CAD build for the part. Positions are in the model's coordinates, mm. A direction names the side the tool comes from. Round coordinates to 2 decimals unless told otherwise and drop trailing zeros. Loops run counter-clockwise (first coordinate to the right, second up) from the corner with the lowest first, then second, coordinate; pieces in that order, holes last. Notation, with made-up numbers: (57, 13.5) - (67, 13.5) arc R27 ccw to (67, 31.5) - close; hole circle Ø8 at (53, 4.5). An arc over 180 degrees is marked (long way). Use one line per item in the form item = value.
from build123d import *

# Parameters (mm, degrees)
SKETCH1_W           = 167
SKETCH1_H           = 106
SKETCH1_R           = 2
BOSS_EXTRUDE1_DEPTH = 3


with BuildPart() as part:
    # Sketch1 → Boss-Extrude1 (new body)
    with BuildSketch(Plane(origin=(0, 0, 0), x_dir=(-1, 0, 0), z_dir=(0, 0, 1))):
        with Locations((-80.5, 50)):
            Rectangle(SKETCH1_W, SKETCH1_H)
        with Locations((-159, 98)):
            Circle(SKETCH1_R, mode=Mode.SUBTRACT)
        with Locations((-2, 98)):
            Circle(SKETCH1_R, mode=Mode.SUBTRACT)
        with Locations((-2, 2)):
            Circle(SKETCH1_R, mode=Mode.SUBTRACT)
        with Locations((-159, 2)):
            Circle(SKETCH1_R, mode=Mode.SUBTRACT)
        with BuildLine():
            Line((-136, 63), (-106, 63))
            ThreePointArc((-106, 63), (-93, 50), (-106, 37))
            Line((-106, 37), (-136, 37))
            ThreePointArc((-136, 37), (-149, 50), (-136, 63))
        make_face(mode=Mode.SUBTRACT)
    extrude(amount=BOSS_EXTRUDE1_DEPTH)


solid = part.part
1) Slice it at B-B (x = 116). Write the cut outline in (y, z), plus the area to 3 significant figures.
Report:
outline = (-103, 0) - (-63, 0) - (-63, 3) - (-103, 3) - close; (-37, 0) - (3, 0) - (3, 3) - (-37, 3) - close
area = 240 mm^2
2) Tool access for faces 1 (the flat face through (82, -51, 0)), 2 (the flat face through (121, -37, 1)): list every direction of +Z, -Z, +X, -X, +Y, -Y with a clear straight run to the whole face (end or side of a thin tool).
Report:
face_1 = -Z, +X, -X, +Y, -Y
face_2 = +Z, -Z
3) Slice it at A-A (y = -50). Write the cut outline in (x, z), plus the area to 3 significant figures.
Report:
outline = (-3, 0) - (93, 0) - (93, 3) - (-3, 3) - close; (149, 0) - (164, 0) - (164, 3) - (149, 3) - close
area = 333 mm^2
4) Two-plate mould, pull along X, no slides. Class faces 3 (the flat face through (164, -49, 1)), 4 (the cylindrical face through (161, -2, 1)), 5 (the flat face through (82, -51, 3)): +X half, -X half, draft (parallel to the pull), parting line (faces both ways), or undercut.
Report:
face_3 = +X half
face_4 = undercut
face_5 = draft
5) Slice it at D-D (z = 1.05). Write the cut outline in (x, y), plus the area to 3 significant figures.
Report:
outline = (-3, -103) - (164, -103) - (164, 3) - (-3, 3) - close; hole circle Ø4 at (2, -98); hole circle Ø4 at (2, -2); hole (106, -63) - (136, -63) arc R13 ccw to (136, -37) - (106, -37) arc R13 ccw to start; hole circle Ø4 at (159, -98); hole circle Ø4 at (159, -2)
area = 16,300 mm^2
6) Drill centre lines: probe 1 along Y at (x, z) = (159, 1.8); probe 2 along X at (y, z) = (-98, 1.55); probe 3 along X at (y, z) = (-50.5, 2.35). Where is each one in solid material? Low to high.
Report:
probe_1 = -103 to -100, -96 to -4, 0 to 3
probe_2 = -3 to 0, 4 to 157, 161 to 164
probe_3 = -3 to 93.01, 148.99 to 164
7) Slice it at C-C (y = -98). Write the cut outline in (x, z).
Report:
outline = (-3, 0) - (0, 0) - (0, 3) - (-3, 3) - close; (4, 0) - (157, 0) - (157, 3) - (4, 3) - close; (161, 0) - (164, 0) - (164, 3) - (161, 3) - close
